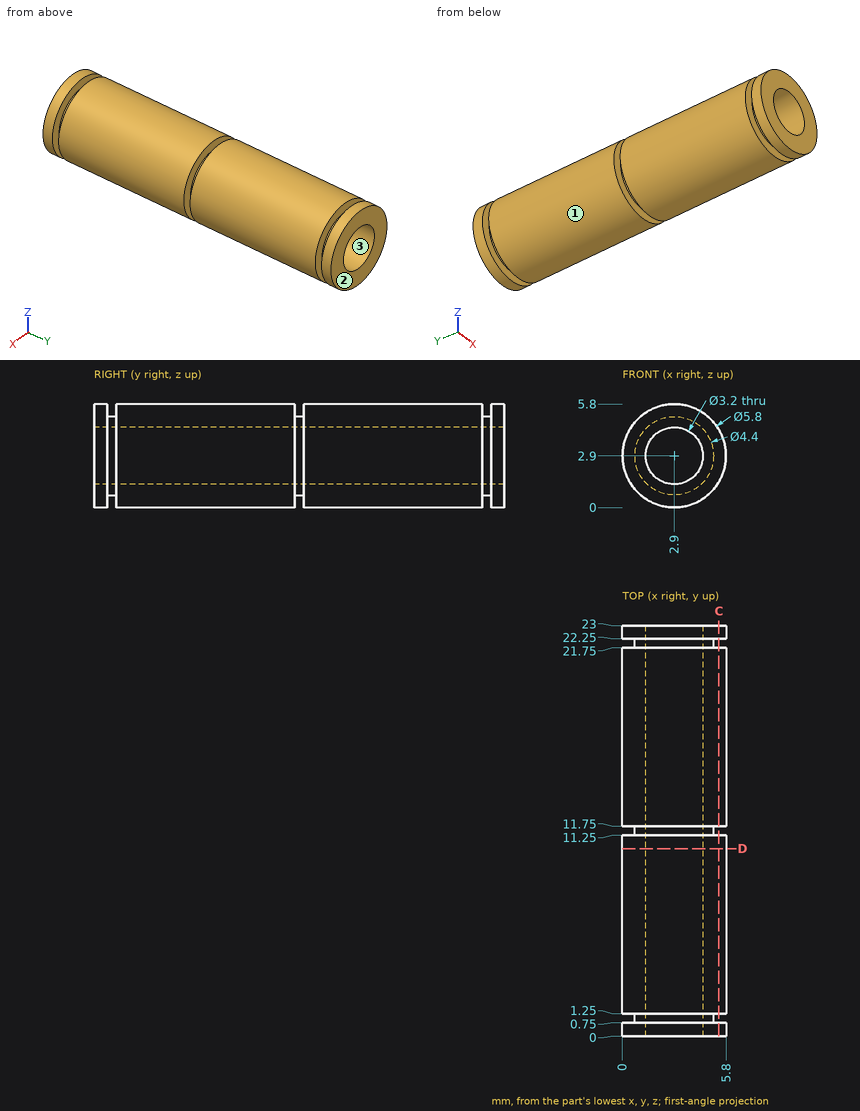
For this review, use the dimensioned drawing (mm, ordinates from the lowest corner) and the shaded views. Coordinates: 2 decimals unless noted, no trailing zeros. Order: outer loops, then holes, each group sorted by start corner. A loop starts at its lowest first (then second) coordinate and runs counter-clockwise, first axis right, second up. Notation, with made-up numbers: (78.25, -27.5) - (108.25, -27.5) arc R17 ccw to (108.25, -0.5) - close; hole circle Ø8 at (42, 51.25). An arc over 180 degrees is marked (long way). Answer as a JSON object with one key per item and string values. Group by question number.
1. We need section C-C on x = 5.4. State the section outline as (y, z) points, then the cut area to 3 significant figures.
2. The part is to be moulded in two halves that separate along X. For the marked faces 1, 2 and 3, say which applies: pulls with the +X half, pulls with the -X half, needs draft (parallel to the pull), parting line crosses it, or undercut.
3. Clearance check with a flat-ended pin moving along its axis: P1, Ø1, axis at x = 0.5, y = 15.5, coming from the -Z side. State where the tip first meets the part, or that it passes through.
4. We need section D-D on y = 10.5. State the section outline as (x, z) points, then the cut area to 3 significant figures.
5. For probe 1 along Y at (x, z) = (1.15, 0.95); probe 2 along Z at (x, y) = (2.9, 13.75), list the stretches that pass through material, from the lowest coordinate up.
Final values:
{
 "1": {"outline": "(0, 1.43) - (0.75, 1.43) - (0.75, 4.37) - (0, 4.37) - close; (1.25, 1.43) - (11.25, 1.43) - (11.25, 4.37) - (1.25, 4.37) - close; (11.75, 1.43) - (21.75, 1.43) - (21.75, 4.37) - (11.75, 4.37) - close; (22.25, 1.43) - (23, 1.43) - (23, 4.37) - (22.25, 4.37) - close", "area": "63.2 mm²"},
 "2": {"face 1": "parting line crosses it", "face 2": "needs draft", "face 3": "undercut"},
 "3": {"P1": "z = 0.71"},
 "4": {"outline": "circle Ø5.8 at (2.9, 2.9); hole circle Ø3.2 at (2.9, 2.9)", "area": "18.4 mm²"},
 "5": {"probe 1": "0 to 0.75, 1.25 to 11.25, 11.75 to 21.75, 22.25 to 23", "probe 2": "0 to 1.3, 4.5 to 5.8"}
}
